Autodesk Inventor part; units mm, degrees
ref_plane "YZ Plane" through (0, 0, 0) normal (1, 0, 0) x (0, 1, 0)
ref_plane "XZ Plane" through (0, 0, 0) normal (0, 1, 0) x (-1, 0, 0)
ref_plane "XY Plane" through (0, 0, 0) normal (0, 0, 1) x (1, 0, 0)
sketch "Sketch1" plane through (0, 0, 0) normal (0, 1, 0) x (-1, 0, 0)
  line L0 (-20.151, 40.9405) -> (15.849, 40.9405)
  line L1 (24.849, 31.9405) -> (24.849, -14.8595)
  line L2 (-0.351, -40.0595) -> (-21.051, -40.0595)
  line L3 (-29.151, -31.9595) -> (-29.151, 31.9405)
  arc A0 (24.849, 31.9405) -> (15.849, 40.9405) centre (15.849, 31.9405) ccw
  arc A1 (-20.151, 40.9405) -> (-29.151, 31.9405) centre (-20.151, 31.9405) ccw
  arc A2 (-29.151, -31.9595) -> (-21.051, -40.0595) centre (-21.051, -31.9595) ccw
  line L4 (24.849, -14.8595) -> (-0.351, -40.0595)
  circle A3 centre (9.082, -4.6389) radius 2.03
  circle A4 centre (-16.112, -29.8255) radius 2.03
  line L5 (15.664, 32.3905) -> (-20.336, 32.3905)
  line L6 (-20.336, 32.3905) -> (-20.336, 22.4905)
  line L7 (-20.336, 22.4905) -> (15.664, 22.4905)
  line L8 (15.664, 22.4905) -> (15.664, 32.3905)
  point P0 (0, 0)
  point P1 (-29.151, 40.9405)
  point P2 (24.849, -40.0595)
  point P3 (24.849, 40.9405)
  point P4 (-29.151, -40.0595)
  dimension "d0" = 9
  dimension "d1" = 8.1
  dimension "d2" = 20.7
  dimension "d3" = 36
  dimension "d4" = 46.8
  dimension "d5" = 9
  dimension "d6" = 63.9
  dimension "d7" = 4.06
  dimension "d8" = 4.06
  dimension "d9" = 15.767
  dimension "d10" = 18.376
  dimension "d11" = 10.234
  dimension "d12" = 13.039
  dimension "d13" = 38.233
  dimension "d14" = 9.9
  dimension "d15" = 36
  dimension "d16" = 8.55
  dimension "d17" = 8.815
  dimension "d18" = 9.185
extrude "Extrusion1" add sketch "Sketch1" along normal blind 9
properties part number "hip hitam"
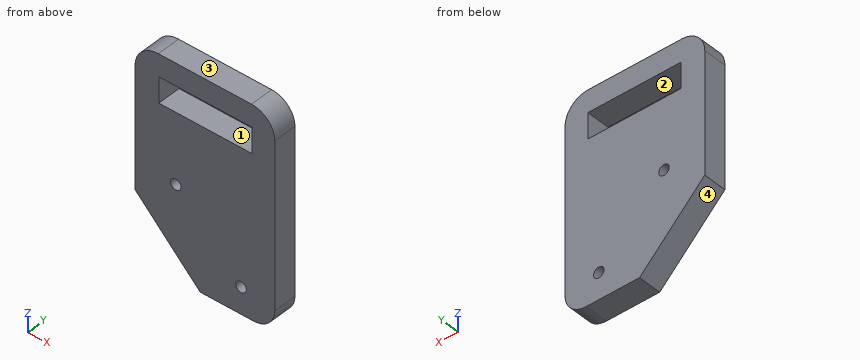
Verification items for the finished model (mm, model axes). Face numbers are marked on the shaded views. Round coordinates to 2 decimals unless told otherwise and drop trailing zeros. Order: outer loops, then holes, each group sorted by start corner. A loop starts at its lowest first (then second) coordinate and runs counter-clockwise, first axis right, second up.
1. Section check B-B on x = 7.5. Record the cut outline in (y, z), then the cut area to 3 significant figures.
Final values:
outline: (0, -40.06) - (9, -40.06) - (9, 22.49) - (0, 22.49) - close; (0, 32.39) - (9, 32.39) - (9, 40.94) - (0, 40.94) - close
area: 640 mm2
2. Thickness scan on L1, parallel to Z at x = 10, y = 2; L2, parallel to Z at x = -8.5, y = 6.5; L3, parallel to Z at x = 15.5, y = 5. Record the ranges inside material, lowest first.
Final values:
L1: z = -40.06 to 22.49, 32.39 to 40.94
L2: z = -31.21 to -6.58, -2.69 to 22.49, 32.39 to 40.94
L3: z = -40.06 to -31.76, -27.89 to 22.49, 32.39 to 40.94
3. Section check A-A on z = 30.5. Record the cut outline in (x, y), then the cut area to 3 significant figures.
Final values:
outline: (-24.85, 0) - (-15.66, 0) - (-15.66, 9) - (-24.85, 9) - close; (20.34, 0) - (29.15, 0) - (29.15, 9) - (20.34, 9) - close
area: 162 mm2
4. Go/stop test with flat-tipped pins: P1, Ø4.5, axis at x = -3, y = 6, coming from the -Z side; P2, Ø2.5, axis at x = 16.11, z = -29.83, coming from the -Y side (3 decimals); P3, Ø3, axis at x = -15.5, y = 6, coming from the -Z side. Record where each tip stops, or that it passes through.
Final values:
P1: stops at z = -38.96
P2: passes through
P3: stops at z = -25.71
5. Section check C-C on x = -9. Record the cut outline in (y, z), then the cut area to 3 significant figures.
Final values:
outline: (0, -30.71) - (9, -30.71) - (9, -6.67) - (0, -6.67) - close; (0, -2.61) - (9, -2.61) - (9, 22.49) - (0, 22.49) - close; (0, 32.39) - (9, 32.39) - (9, 40.94) - (0, 40.94) - close
area: 519 mm2
6. Release check for a two-part mould opening along Z. For the marked faces 1, 2, 3 and 4 record: +Z half, -Z half, draft (parallel to the pull), parting line (faces both ways), or undercut.
Final values:
face 1: undercut
face 2: undercut
face 3: +Z half
face 4: -Z half
7. Section check D-D on y = 7.25. Record the cut outline in (x, z).
Final values:
outline: (-24.85, -14.86) - (0.35, -40.06) - (21.05, -40.06) arc R8.1 ccw to (29.15, -31.96) - (29.15, 31.94) arc R9 ccw to (20.15, 40.94) - (-15.85, 40.94) arc R9 ccw to (-24.85, 31.94) - close; hole (-15.66, 22.49) - (20.34, 22.49) - (20.34, 32.39) - (-15.66, 32.39) - close; hole circle Ø4.06 at (-9.08, -4.64); hole circle Ø4.06 at (16.11, -29.83)
